Geometry check sheet. Reference: drawing and pictorial views, mm from the part's lowest x, y, z. A direction names the side the tool comes from. Give positions to 0.01 mm unless a question says otherwise; leave off trailing zeros. Write each loop counter-clockwise with the first axis right and the second up, starting at its lowest first coordinate (ties: lowest second). Pieces come first, ordered by that corner, then holes.
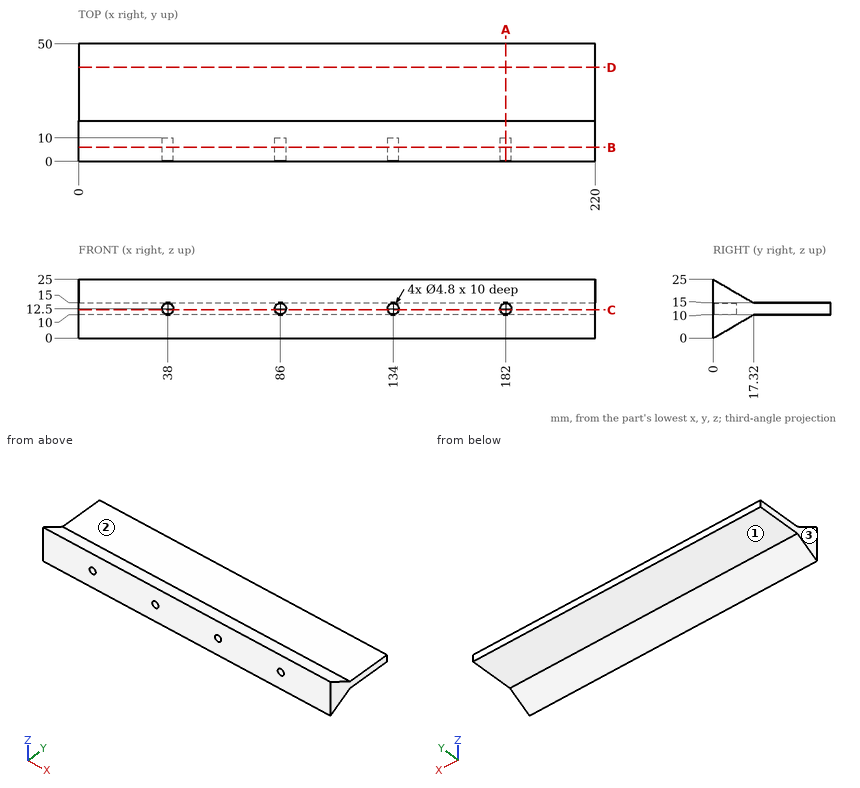
Item 1: Sectioned sample at A-A on x = 182. Record the cut outline in (y, z).
Answer key:
outline: (0, 0) - (17.32, 10) - (50, 10) - (50, 15) - (17.32, 15) - (0, 25) - (0, 14.9) - (10, 14.9) - (10, 10.1) - (0, 10.1) - close
Item 2: Sectioned sample at C-C on z = 12. Record the cut outline in (x, y).
Answer key:
outline: (0, 0) - (35.65, 0) - (35.65, 10) - (40.35, 10) - (40.35, 0) - (83.65, 0) - (83.65, 10) - (88.35, 10) - (88.35, 0) - (131.65, 0) - (131.65, 10) - (136.35, 10) - (136.35, 0) - (179.65, 0) - (179.65, 10) - (184.35, 10) - (184.35, 0) - (220, 0) - (220, 50) - (0, 50) - close
Item 3: Sectioned sample at B-B on y = 6. Record the cut outline in (x, z) (1 decimal), then the cut area to 3 significant figures.
Answer key:
outline: (0, 3.5) - (220, 3.5) - (220, 21.5) - (0, 21.5) - close; hole circle Ø4.8 at (38, 12.5); hole circle Ø4.8 at (86, 12.5); hole circle Ø4.8 at (134, 12.5); hole circle Ø4.8 at (182, 12.5)
area: 3,900 mm2
Item 4: Sectioned sample at D-D on y = 40. Record the cut outline in (x, z), then the cut area to 3 significant figures.
Answer key:
outline: (0, 10) - (220, 10) - (220, 15) - (0, 15) - close
area: 1,100 mm2
Item 5: Scan lines: line 1 along X through (y, z) = (6, 12.5); line 2 along Z through (x, y) = (59.5, 33); line 3 along Z through (x, y) = (86, 7.75) (1 decimal). Record each from-to range of solid material in increasing order.
Answer key:
line 1: x = 0 to 35.6, 40.4 to 83.6, 88.4 to 131.6, 136.4 to 179.6, 184.4 to 220
line 2: z = 10 to 15
line 3: z = 4.5 to 10.1, 14.9 to 20.5
Item 6: Depth check by flat-ended pin: pin 1 (4 mm diameter, centred on x = 86, z = 12.5, fed in from -Y); pin 2 (4 mm diameter, centred on x = 40, y = 25, fed in from +Z); pin 3 (3 mm diameter, centred on x = 119.5, y = 34.5, fed in from -Z). Enter the tip coordinate at first touch or a pass-through.
Answer key:
pin 1: stops at y = 10
pin 2: stops at z = 15
pin 3: stops at z = 10
Item 7: Set-up check for the marked faces 1, 2 and 3: record each of +Z, -Z, +X, -X, +Y, -Y from which the full face is reachable in a straight line by a thin tool's end or side.
Answer key:
face 1: -Z, +X, -X, +Y
face 2: +Z, +X, -X, +Y
face 3: +Z, -Z, -X, +Y, -Y
